```python
from build123d import *

# Parameters (mm, degrees)
SKETCH1_R           = 10
SKETCH1_R_2         = 3.025
BOSS_EXTRUDE1_DEPTH = 4.25
CUT_EXTRUDE1_DEPTH  = 2
SKETCH4_R           = 1.125
CUT_EXTRUDE2_DEPTH  = 15.320003492
SKETCH5_R           = 10
SKETCH5_R_2         = 1.125
SKETCH5_R_3         = 3.025
BOSS_EXTRUDE2_DEPTH = 4.25
SHELL1_T            = -1


with BuildPart() as part:
    # Sketch1 → Boss-Extrude1 (new body)
    with BuildSketch(Plane(origin=(0, 0, 0), x_dir=(1, 0, 0), z_dir=(0, 1, 0))):
        with Locations(Location((0, 0, 0), (0, 0, 270))):
            Circle(SKETCH1_R)
        with Locations(Location((0, 0, 0), (0, 0, 270))):
            Circle(SKETCH1_R_2, mode=Mode.SUBTRACT)
    extrude(amount=BOSS_EXTRUDE1_DEPTH)

    # Sketch3 → Cut-Extrude1 (cut)
    with BuildSketch(Plane.XZ):
        Polygon((7, 2.309401077), (5, 1.154700538), (5, -1.154700538), (7, -2.309401077), (9, -1.154700538), (9, 1.154700538), align=None)
        Polygon((-2.309401077, 7), (-1.154700538, 5), (1.154700538, 5), (2.309401077, 7), (1.154700538, 9), (-1.154700538, 9), align=None)
        Polygon((2.309401077, -7), (1.154700538, -5), (-1.154700538, -5), (-2.309401077, -7), (-1.154700538, -9), (1.154700538, -9), align=None)
        Polygon((-7, -2.309401077), (-5, -1.154700538), (-5, 1.154700538), (-7, 2.309401077), (-9, 1.154700538), (-9, -1.154700538), align=None)
    extrude(amount=-CUT_EXTRUDE1_DEPTH, mode=Mode.SUBTRACT)

    # Sketch4 → Cut-Extrude2 (cut, through all)
    with BuildSketch(Plane.XZ.offset(-2)):
        with Locations(Location((0, -7, 0), (0, 0, 270))):
            Circle(SKETCH4_R)
        with Locations(Location((0, 7, 0), (0, 0, 270))):
            Circle(SKETCH4_R)
        with Locations(Location((7, 0, 0), (0, 0, 270))):
            Circle(SKETCH4_R)
        with Locations(Location((-7, 0, 0), (0, 0, 270))):
            Circle(SKETCH4_R)
    extrude(amount=-CUT_EXTRUDE2_DEPTH, mode=Mode.SUBTRACT)

    # Sketch5 → Boss-Extrude2 (add)
    with BuildSketch(Plane.XZ):
        with Locations(Location((0, 0, 0), (0, 0, 90))):
            Circle(SKETCH5_R)
        with Locations(Location((7, 0, 0), (0, 0, 270))):
            Circle(SKETCH5_R_2, mode=Mode.SUBTRACT)
        with Locations(Location((0, -7, 0), (0, 0, 270))):
            Circle(SKETCH5_R_2, mode=Mode.SUBTRACT)
        with Locations(Location((-7, 0, 0), (0, 0, 270))):
            Circle(SKETCH5_R_2, mode=Mode.SUBTRACT)
        with Locations(Location((0, 7, 0), (0, 0, 270))):
            Circle(SKETCH5_R_2, mode=Mode.SUBTRACT)
        with Locations(Location((0, 0, 0), (0, 0, 90))):
            Circle(SKETCH5_R_3, mode=Mode.SUBTRACT)
    extrude(amount=-BOSS_EXTRUDE2_DEPTH)

    # Shell1
    shell1_openings = [part.faces().sort_by_distance(p)[0] for p in [
        (0, 0, -9.717157288),
    ]]
    offset(amount=SHELL1_T, openings=shell1_openings)


solid = part.part
```
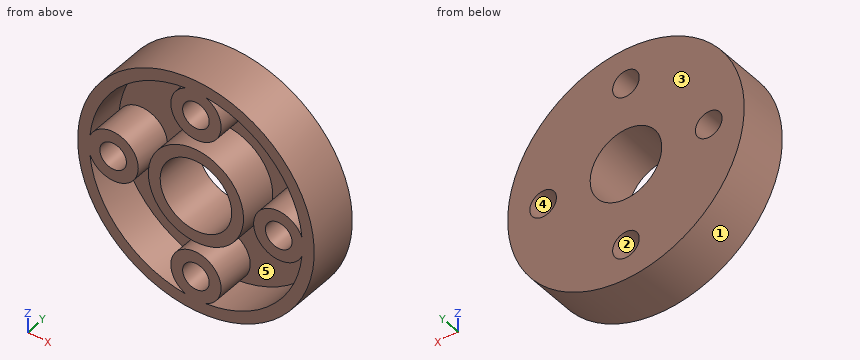
Check sheet for the modelled part. Datum: model origin and axes. Units: mm. Face numbers are marked on the shaded views. A direction names the side the tool comes from. Coordinates: 2 decimals unless noted, no trailing zeros. Write each loop counter-clockwise with the first axis right and the second up, starting at its lowest first coordinate (ties: lowest second). Pieces come first, ordered by that corner, then holes. Notation, with made-up numbers: M -6,84.25 L 13,84.25 A25 cw 13,104.25 Z; hole C 34.25,70.25 d7. An arc over 180 degrees is marked long. Use one line per item in the form item = value.
Item 1: Sectioned sample at D-D, the plane z = -7.5. Record the cut outline in (x, y), and give its area (3 significant figures).
Answer below:
outline = M -6.61,0 L -4.97,0 L -4.97,3.25 L -2.07,3.25 L -2.07,0 L -1.01,0 L -1.01,4.25 L -6.61,4.25 Z; M 1.01,0 L 2.07,0 L 2.07,3.25 L 4.97,3.25 L 4.97,0 L 6.61,0 L 6.61,4.25 L 1.01,4.25 Z
area = 28.7 mm^2
Item 2: Sectioned sample at A-A, the plane z = 0. Record the cut outline in (x, y) (3 decimals).
Answer below:
outline = M -10,0 L -8.125,0 L -8.125,4.25 L -10,4.25 Z; M -5.875,0 L -4.875,0 L -4.875,3.25 L -4.025,3.25 L -4.025,0 L -3.025,0 L -3.025,4.25 L -5.875,4.25 Z; M 3.025,0 L 4.025,0 L 4.025,3.25 L 4.875,3.25 L 4.875,0 L 5.875,0 L 5.875,4.25 L 3.025,4.25 Z; M 8.125,0 L 10,0 L 10,4.25 L 8.125,4.25 Z
Item 3: Sectioned sample at C-C, the plane x = 7. Record the cut outline in (y, z) (3 decimals).
Answer below:
outline = M 0,-7.141 L 4.25,-7.141 L 4.25,-1.125 L 0,-1.125 L 0,-2.125 L 3.25,-2.125 L 3.25,-5.657 L 0,-5.657 Z; M 0,1.125 L 4.25,1.125 L 4.25,7.141 L 0,7.141 L 0,5.657 L 3.25,5.657 L 3.25,2.125 L 0,2.125 Z
Item 4: Set-up check for the marked faces 4 and 5: record each of +Z, -Z, +X, -X, +Y, -Y from which the full face is reachable in a straight line by a thin tool's end or side.
Answer below:
face_4 = +Y, -Y
face_5 = -Y
Item 5: Material ranges on L1, parallel to Z at x = 6.25, y = 1.6; L2, parallel to Z at x = 0.25, y = 3.75; L3, parallel to X at y = 2.75, z = 2.25, recorded low to high. Write a range as from..to.
Answer below:
L1 = -7.81..-6.48, -1.99..-0.84, 0.84..1.99, 6.48..7.81
L2 = -10..-8.1, -5.9..-3.01, 3.01..5.9, 8.1..10
L3 = -9.74..-8.71, -3.34..-2.02, 2.02..3.34, 8.71..9.74
Item 6: Gauge pin test, flat ends, axial feed: pin 1 Ø1.5 at (x, y) = (-6, 1.5) entering from +Z; pin 2 Ø1.5 at (y, z) = (2.5, 5) entering from -X; pin 3 Ø1.8 at (x, z) = (0, -7) entering from -Y. Record the tip position at first contact, or that the pin passes through.
Answer below:
pin_1 = 8.51
pin_2 = -9.05
pin_3 = through
Item 7: Release check for a two-part mould opening along Z. For the marked faces 1, 2 and 3 record: pulls with the +Z half, pulls with the -Z half, needs draft (parallel to the pull), parting line crosses it, or undercut.
Answer below:
face_1 = parting line crosses it
face_2 = undercut
face_3 = needs draft
Item 8: Sectioned sample at B-B, the plane y = 3.55. Record the cut outline in (x, z) (3 decimals), and give its area (3 significant figures).
Answer below:
outline = C 0,0 d20; hole C -7,0 d2.25; hole C 0,0 d6.05; hole C 0,-7 d2.25; hole C 0,7 d2.25; hole C 7,0 d2.25
area = 270 mm^2
